Build history of the part. All positions in model axes, mm. A direction names the side the tool comes from. Give positions to 0.01 mm unless a question says otherwise; leave off trailing zeros. Order: outer loops, then holes, each group sorted by start corner. A loop starts at its lowest first (then second) coordinate and runs counter-clockwise, first axis right, second up. Notation, with made-up numbers: (23, -29.75) - (59, -29.75) arc R8 ccw to (59, -18.75) - close; hole circle Ø1 at (53.5, 30). An arc over 180 degrees is marked (long way). One line per item, written item: value.
```python
from build123d import *

# Parameters (mm, degrees)
F1_DEPTH = 4


with BuildPart() as f1:
    # F0 (on Top) → F1 (new body)
    with BuildSketch(Plane.XY):
        with BuildLine():
            Line((-2.5, 15), (-2.5, 0))
            Line((-2.5, 0), (0, 0))
            Line((0, 0), (0, 39.919411))
            Line((0, 39.919411), (-5, 39.919411))
            Line((-5, 39.919411), (-5, 28.919411))
            ThreePointArc((-5, 28.919411), (-3.129961, 22.071068), (-2.5, 15))
        make_face()
    extrude(amount=F1_DEPTH)

    # F2: F1 across face


with BuildPart() as f1_1:
    add(f1.part)
    add(f1.part.mirror(Plane(origin=(0, 19.959705, 2), x_dir=(0, 1, 0), z_dir=(1, 0, 0))))

    # F3: F1 across face


with BuildPart() as f1_2:
    add(f1_1.part)
    add(f1_1.part.mirror(Plane(origin=(0, 0, 2), x_dir=(1, 0, 0), z_dir=(0, -1, 0))))


solid = f1_2.part
```
(1) Drill centre lines: line 1 (X direction, y = 3, z = 2.1); line 2 (X direction, y = -27, z = 1.8). Where is each one in solid material? Low to high.
Completed:
line 1: -2.5 to 2.5
line 2: -4.34 to 4.34
(2) Slice it at B-B, the plane z = 0.95. Give the cut face in (x, y).
Completed:
outline: (-5, -39.92) - (5, -39.92) - (5, -28.92) arc R40 cw to (2.5, -15) - (2.5, 15) arc R40 cw to (5, 28.92) - (5, 39.92) - (-5, 39.92) - (-5, 28.92) arc R40 cw to (-2.5, 15) - (-2.5, -15) arc R40 cw to (-5, -28.92) - close
(3) Slice it at D-D, the plane y = -21. Give the cut face in (x, z).
Completed:
outline: (-2.95, 0) - (2.95, 0) - (2.95, 4) - (-2.95, 4) - close
(4) 3-axis set-ups, long thin cutter, end or side, ignore diameter. For faces 1 (the face through (3.148, -22.169, 1.972)), 2 (the face through (0, -1, 4)), 3 (the face through (-2.5, 0, 2)): which of +Z, -Z, +X, -X, +Y, -Y reach the whole face in a straight line?
Completed:
face 1: +Z, -Z, +X
face 2: +Z, +X, -X, +Y, -Y
face 3: +Z, -Z, -X
(5) Pull direction Y, two halves, no side cores. Call faces 4 (the face through (-3.148, -22.169, 1.972)), 5 (the face through (5, 34, 2)), 6 (the face through (0, 39.919, 2)), 7 (the face through (-3.148, 22.169, 1.972)): +Y half, -Y half, draft (parallel to the pull), parting line (faces both ways), or undercut.
Completed:
face 4: undercut
face 5: draft
face 6: +Y half
face 7: undercut
(6) Pin check, flat tips, straight feed: P1, Ø1.5, axis at y = 12.5, z = 1.5, coming from the +X side; P2, Ø5, axis at x = -3.5, y = 21.5, coming from the -Z side; P3, Ø1, axis at x = -3.5, y = -12.5, coming from the +Z side; P4, Ø1.2, axis at y = -3, z = 2, coming from the -X side. Stop position of each tip, or through.
Completed:
P1: x = 2.5
P2: z = 0
P3: through
P4: x = -2.5
(7) Slice it at A-A, the plane x = -3.25. Give the cut face in (y, z), and give its area (3 significant figures).
Completed:
outline: (-39.92, 0) - (-22.71, 0) - (-22.71, 4) - (-39.92, 4) - close; (22.71, 0) - (39.92, 0) - (39.92, 4) - (22.71, 4) - close
area: 138 mm²
(8) Slice it at C-C, the plane y = -4. Give the cut face in (x, z).
Completed:
outline: (-2.5, 0) - (2.5, 0) - (2.5, 4) - (-2.5, 4) - close
